Verification items for this drawing (mm, ordinates from the low corner). A direction names the side the tool comes from. Round coordinates to 2 decimals unless told otherwise and drop trailing zeros. Loops run counter-clockwise (first coordinate to the right, second up) from the corner with the lowest first, then second, coordinate; pieces in that order, holes last. Notation, with made-up numbers: (-19, 3) - (21, 3) arc R28 cw to (21, 33) - close; hole circle Ø4 at (58, -14). An arc over 180 degrees is marked (long way). Write item = value, one per line.
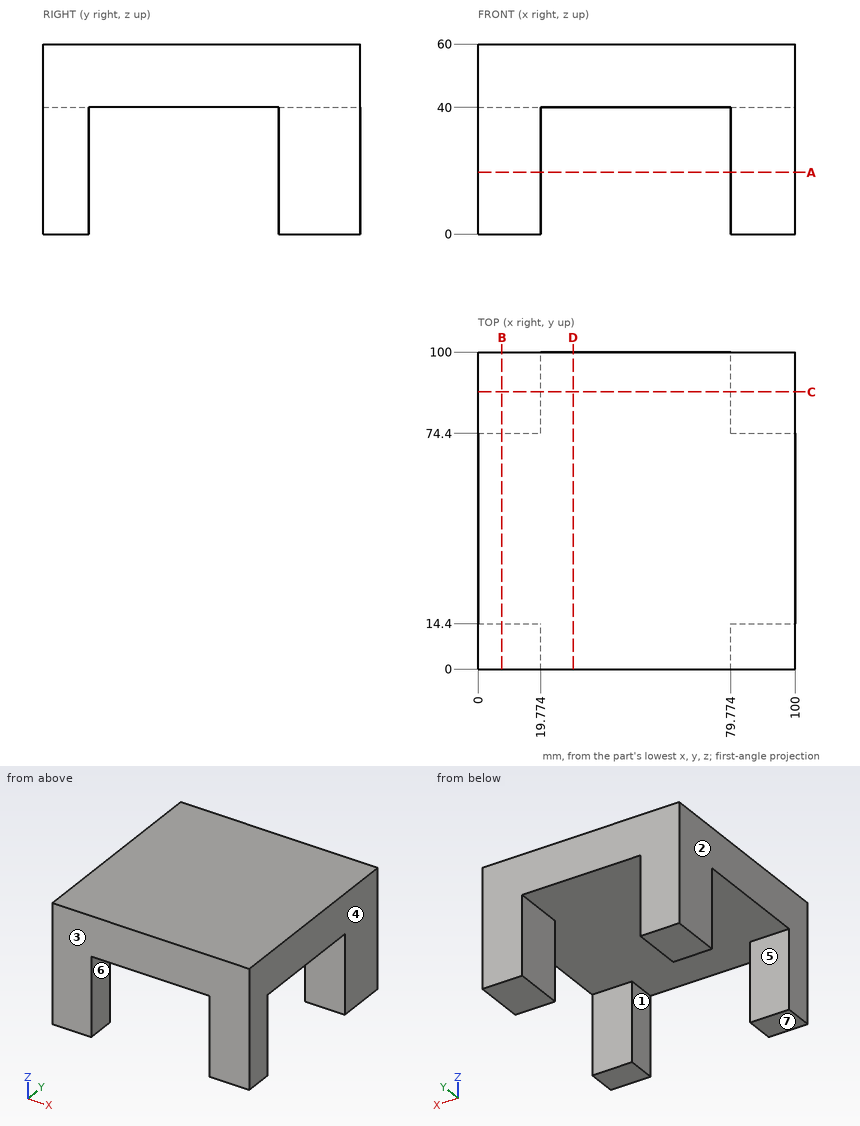
(1) Section check D-D (x = 30). Enter the section's corners in (y, z), then the cut area to 3 significant figures.
Answers follow:
outline = (0, 40) - (100, 40) - (100, 60) - (0, 60) - close
area = 2,000 mm²
(2) Mould release check, pull along X, two halves, no side actions. Record for the marked faces 1, 2, 3 and 4: pulls with the +X half, pulls with the -X half, needs draft (parallel to the pull), parting line crosses it, or undercut.
Answers follow:
face_1 = undercut
face_2 = pulls with the -X half
face_3 = needs draft
face_4 = pulls with the +X half
(3) Section check B-B (x = 7.5). Enter the section's corners in (y, z).
Answers follow:
outline = (0, 0) - (14.4, 0) - (14.4, 40) - (74.4, 40) - (74.4, 0) - (100, 0) - (100, 60) - (0, 60) - close
(4) Gauge pin test, flat end, axial feed: pin 1 (10 mm diameter, centred on x = 32.5, y = 70.5, fed in from -Z). Record the tip position at first contact, or that the pin passes through.
Answers follow:
pin_1 = 40
(5) Set-up check for the marked faces 5, 6 and 7: record each of +Z, -Z, +X, -X, +Y, -Y from which the full face is reachable in a straight line by a thin tool's end or side.
Answers follow:
face_5 = -Z, +X, -X
face_6 = -Z, +Y, -Y
face_7 = -Z, +X, -X, +Y, -Y
(6) Section check C-C (y = 87.5). Enter the section's corners in (x, z), then the cut area to 3 significant figures.
Answers follow:
outline = (0, 0) - (19.77, 0) - (19.77, 40) - (79.77, 40) - (79.77, 0) - (100, 0) - (100, 60) - (0, 60) - close
area = 3,600 mm²
(7) Section check A-A (z = 19.5). Enter the section's corners in (x, y).
Answers follow:
outline = (0, 0) - (19.77, 0) - (19.77, 14.4) - (0, 14.4) - close; (0, 74.4) - (19.77, 74.4) - (19.77, 100) - (0, 100) - close; (79.77, 0) - (100, 0) - (100, 14.4) - (79.77, 14.4) - close; (79.77, 74.4) - (100, 74.4) - (100, 100) - (79.77, 100) - close
(8) Scan lines: L1, parallel to Y at x = 17, z = 39; L2, parallel to X at y = 82, z = 25; L3, parallel to Z at x = 53, y = 16.5. Record each from-to range of solid material in increasing order. Write a range as [from, to].
Answers follow:
L1 = [0, 14.4], [74.4, 100]
L2 = [0, 19.77], [79.77, 100]
L3 = [40, 60]
